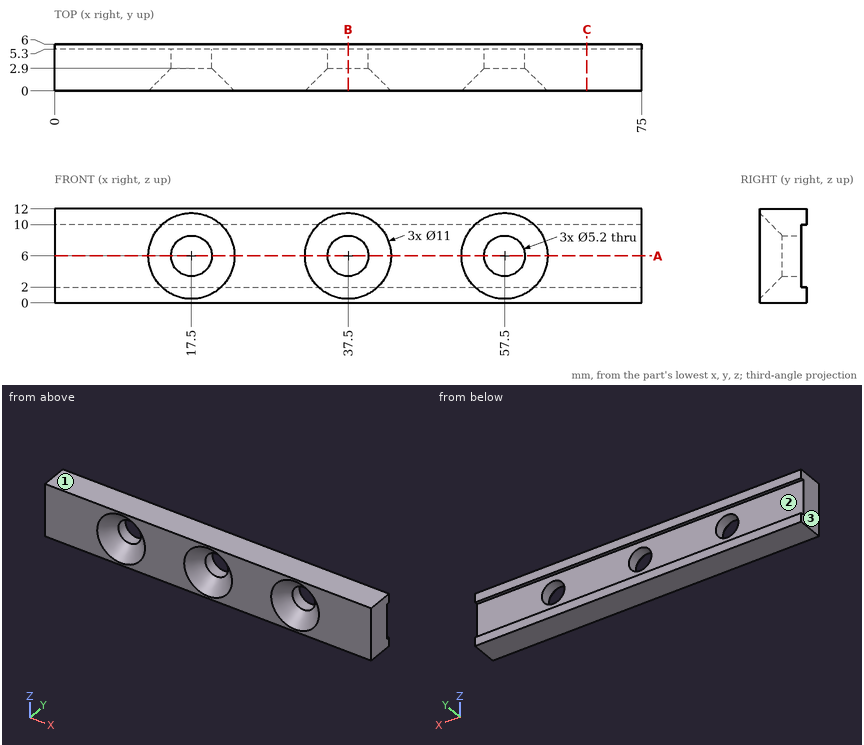
Verification items for this drawing (mm, ordinates from the low corner). Give positions to 0.01 mm unless a question says otherwise; leave off trailing zeros. Loops run counter-clockwise (first coordinate to the right, second up) from the corner with the lowest first, then second, coordinate; pieces in that order, holes last. Notation, with made-up numbers: M 88,-23.75 L 112,-23.75 A10 ccw 112,-16.75 Z; hole C 75,66 d2. An arc over 180 degrees is marked long. Return JSON: item names as keys, results as strings. Group by question number.
1. Cross-section at A-A on z = 6. Record the boundary of the cut face in (x, y), plus the area to 3 significant figures.
2. Go/stop test with flat-tipped pins: pin 1 (5 mm diameter, centred on x = 9, z = 7, fed in from +Y); pin 2 (6 mm diameter, centred on x = 37.5, z = 6, fed in from -Y); pin 3 (5 mm diameter, centred on x = 37, z = 5, fed in from -Y); pin 4 (0.8 mm diameter, centred on x = 52.5, y = 5.5, fed in from -Z). Record where each tip stops, or that it passes through.
3. Thickness scan on L1, parallel to X at y = 3.9, z = 6; L2, parallel to Z at x = 37.5, y = 3.7; L3, parallel to X at y = 1.65, z = 2.5. Record the ranges inside material, lowest first.
4. Mould release check, pull along Z, two halves, no side actions. Record for the marked faces 1, 2 and 3: released by +Z, released by -Z, zero draft, split by the parting line, or undercut.
5. Cross-section at C-C on x = 68. Record the boundary of the cut face in (y, z).
6. Cross-section at B-B on x = 37.5. Record the boundary of the cut face in (y, z), plus the area to 3 significant figures.
Return value:
{
 "1": {"outline": "M 0,0 L 12,0 L 14.9,2.9 L 14.9,5.3 L 0,5.3 Z; M 20.1,2.9 L 23,0 L 32,0 L 34.9,2.9 L 34.9,5.3 L 20.1,5.3 Z; M 40.1,2.9 L 43,0 L 52,0 L 54.9,2.9 L 54.9,5.3 L 40.1,5.3 Z; M 60.1,2.9 L 63,0 L 75,0 L 75,5.3 L 60.1,5.3 Z", "area": "290 mm^2"},
 "2": {"pin 1": "y = 5.3", "pin 2": "y = 2.5", "pin 3": "y = 1.88", "pin 4": "z = 0"},
 "3": {"L1": "0 to 14.9, 20.1 to 34.9, 40.1 to 54.9, 60.1 to 75", "L2": "0 to 3.4, 8.6 to 12", "L3": "0 to 15.9, 19.1 to 35.9, 39.1 to 55.9, 59.1 to 75"},
 "4": {"face 1": "released by +Z", "face 2": "undercut", "face 3": "zero draft"},
 "5": {"outline": "M 0,0 L 6,0 L 6,2 L 5.3,2 L 5.3,10 L 6,10 L 6,12 L 0,12 Z"},
 "6": {"outline": "M 0,0 L 6,0 L 6,2 L 5.3,2 L 5.3,3.4 L 2.9,3.4 L 0,0.5 Z; M 0,11.5 L 2.9,8.6 L 5.3,8.6 L 5.3,10 L 6,10 L 6,12 L 0,12 Z", "area": "30.4 mm^2"}
}
